Autodesk Inventor part; units mm, degrees
ref_plane "YZ Plane" through (0, 0, 0) normal (1, 0, 0) x (0, 1, 0)
ref_plane "XZ Plane" through (0, 0, 0) normal (0, 1, 0) x (-1, 0, 0)
ref_plane "XY Plane" through (0, 0, 0) normal (0, 0, 1) x (1, 0, 0)
sketch "Sketch1" plane through (0, 0, 0) normal (1, 0, 0) x (0, 1, 0)
  line L0 (95.25, -63.5) -> (7.9502, -63.5) construction
  arc A0 (95.25, -63.5) -> (127, -31.75) centre (95.25, -31.75) ccw construction
  circle A1 centre (104.9083, -202.0677) radius 25.4 construction
  circle A2 centre (104.9083, -202.0677) radius 14.2875
  circle A3 centre (154.8209, -171.8196) radius 25.4 construction
  circle A4 centre (154.8209, -171.8196) radius 14.2875
  circle A5 centre (250.0002, -47.5843) radius 22.225 construction
  circle A6 centre (250.0002, -47.5843) radius 25.4 construction
  circle A7 centre (250.0002, -47.5843) radius 14.2875
  circle A8 centre (154.8209, -171.8196) radius 22.225 construction
  circle A9 centre (104.9083, -202.0677) radius 22.225 construction
  circle A10 centre (25.4, -99.06) radius 25.4 construction
  circle A11 centre (25.4, -99.06) radius 23.8125 construction
  line L1 (25.4, -73.66) -> (25.4, -63.5) construction
  circle A12 centre (219.8086, -102.3786) radius 25.4 construction
  circle A13 centre (219.8086, -102.3786) radius 22.225 construction
  circle A14 centre (219.8086, -102.3786) radius 14.2875
  circle A15 centre (63.172, -79.375) radius 6.477 construction
  circle A16 centre (25.4, -99.06) radius 14.2875
  circle A17 centre (63.172, -79.375) radius 3.2512 construction
  circle A18 centre (166.1747, -221.0415) radius 3.2512 construction
  line L2 (219.8086, -102.3786) -> (154.8209, -171.8196) construction
  line L3 (154.8209, -171.8196) -> (104.9083, -202.0677) construction
  circle A19 centre (166.1747, -221.0415) radius 6.4262 construction
  circle A20 centre (63.172, -79.375) radius 6.35 construction
  circle A21 centre (25.4, -99.06) radius 22.225 construction
  line L4 (3.175, -99.06) -> (3.175, -68.2752) construction
  arc A22 (166.1747, -227.4677) -> (170.1786, -226.0679) centre (166.1747, -221.0415) ccw
  arc A23 (3.175, -99.06) -> (35.6756, -118.7669) centre (25.4, -99.06) ccw construction
  arc A24 (7.9502, -63.5) -> (3.175, -68.2752) centre (7.9502, -68.2752) ccw construction
  line L5 (232.868, -28.832) -> (267.1324, -66.3365) construction
  circle A25 centre (232.868, -28.832) radius 2.4257
  circle A26 centre (267.1324, -66.3365) radius 2.4257 construction
  circle A27 centre (232.868, -28.832) radius 6.35 construction
  circle A28 centre (267.1324, -66.3365) radius 6.35 construction
  line L6 (219.8086, -102.3786) -> (237.1646, -83.8332) construction
  line L7 (219.8086, -102.3786) -> (202.4526, -120.9239) construction
  circle A29 centre (237.1646, -83.8332) radius 2.4257 construction
  circle A30 centre (202.4526, -120.9239) radius 2.4257 construction
  circle A31 centre (172.1769, -153.2743) radius 2.4257 construction
  circle A32 centre (133.0985, -184.9838) radius 2.4257 construction
  arc A33 (83.3089, -196.8314) -> (103.7686, -224.2634) centre (104.9083, -202.0677) ccw
  circle A34 centre (9.525, -79.2321) radius 2.4257
  circle A35 centre (9.525, -79.2321) radius 6.35 construction
  line L8 (9.525, -79.2321) -> (41.275, -118.8879) construction
  circle A36 centre (41.275, -118.8879) radius 2.4257 construction
  circle A37 centre (41.275, -118.8879) radius 5.6007 construction
  line L9 (7.9502, -63.5) -> (95.25, -63.5) construction
  arc A38 (95.25, -63.5) -> (127, -31.75) centre (95.25, -31.75) ccw construction
  line L10 (166.1747, -227.4677) -> (103.7686, -224.2634)
  line L11 (104.9083, -202.0677) -> (83.1859, -215.2319) construction
  line L12 (127, -31.75) -> (127, -26.9595) construction
  circle A39 centre (133.0985, -184.9838) radius 5.6007 construction
  circle A40 centre (277.7476, -102.0288) radius 30 construction
  circle A41 centre (277.7476, -102.0288) radius 25.4 construction
  circle A42 centre (277.7476, -102.0288) radius 9.525
  circle A43 centre (219.8086, -102.3786) radius 19.05 construction
  circle A44 centre (227.4601, -139.7023) radius 19.05 construction
  circle A45 centre (227.4601, -139.7023) radius 14.2875
  line L13 (247.7482, -102.2099) -> (245.2082, -102.2252) construction
  line L14 (170.1786, -226.0679) -> (296.4391, -125.4942)
  arc A46 (296.4391, -125.4942) -> (303.3752, -86.4331) centre (277.7476, -102.0288) ccw
  circle A47 centre (219.8086, -102.3786) radius 30.48 construction
  circle A48 centre (277.7476, -102.0288) radius 30.48 construction
  circle A49 centre (248.6408, -79.4624) radius 3.81 construction
  line L15 (251.6519, -81.7968) -> (253.6592, -83.3531) construction
  line L16 (245.6582, -81.833) -> (243.6698, -83.4134) construction
  circle A50 centre (248.6408, -79.4624) radius 2.3812 construction
  circle A51 centre (248.9154, -124.945) radius 3.81 construction
  circle A52 centre (248.9154, -124.945) radius 2.3876 construction
  line L17 (251.898, -122.5744) -> (253.8865, -120.9939) construction
  line L18 (245.9043, -122.6105) -> (243.897, -121.0542) construction
  line L19 (248.6408, -75.6524) -> (248.6408, -72.9479) construction
  line L20 (219.8086, -102.3786) -> (219.8086, -88.0911) construction
  line L21 (131.7752, -22.1843) -> (250.0002, -22.1843)
  line L22 (271.6983, -34.3799) -> (303.3752, -86.4331)
  arc A53 (271.6983, -34.3799) -> (250.0002, -22.1843) centre (250.0002, -47.5843) ccw
  arc A54 (131.7752, -22.1843) -> (127, -26.9595) centre (131.7752, -26.9595) ccw
  circle A55 centre (146.08, -220.0775) radius 6.35 construction
  circle A56 centre (146.08, -220.0775) radius 2.4257
  circle A57 centre (253.6387, -151.4689) radius 6.35 construction
  circle A58 centre (253.6387, -151.4689) radius 2.4257
  circle A59 centre (209.9304, -186.285) radius 6.35 construction
  circle A60 centre (209.9304, -186.285) radius 2.4257
  circle A61 centre (123.7263, -57.0623) radius 6.35 construction
  circle A62 centre (123.7263, -57.0623) radius 2.4257
  circle A63 centre (281.6771, -62.9926) radius 6.35 construction
  circle A64 centre (281.6771, -62.9926) radius 2.4257
  line L23 (123.7263, -57.0623) -> (232.868, -28.832) construction
  line L24 (232.868, -28.832) -> (281.6771, -62.9926) construction
  line L25 (281.6771, -62.9926) -> (253.6387, -151.4689) construction
  line L26 (253.6387, -151.4689) -> (209.9304, -186.285) construction
  line L27 (209.9304, -186.285) -> (146.08, -220.0775) construction
  line L28 (146.08, -220.0775) -> (9.525, -79.2321) construction
  line L29 (123.7263, -57.0623) -> (9.525, -79.2321) construction
  line L30 (117.555, -55.5662) -> (83.3089, -196.8314)
  arc A65 (118.9802, -52.8436) -> (127, -26.9595) centre (94.4844, -31.0695) ccw
  arc A66 (118.9802, -52.8436) -> (117.555, -55.5662) centre (123.7263, -57.0623) ccw
  point P0 (180.2209, -171.8196)
  point P1 (172.6009, -221.0415)
  point P2 (104.9083, -227.4677)
  point P3 (127, -22.1843)
  point P4 (250.0002, -47.5843)
  point P5 (0, 0)
  point P6 (95.25, -63.5)
  dimension "d4" = 31.75
  dimension "d17" = 50.8
  dimension "d18" = 1.5875
  dimension "d21" = 12.954
  dimension "d22" = 28.575
  dimension "d23" = 6.5024
  dimension "d26" = 130.175
  dimension "d27" = 15.875
  dimension "d28" = 6.5024
  dimension "d29" = 143.1895
  dimension "d41" = 3.175
  dimension "d42" = 12.7
  dimension "d43" = 10.16
  dimension "d44" = 50.8
  dimension "d45" = 3.175
  dimension "d46" = 44.45
  dimension "d53" = 3.175
  dimension "d55" = 4.7752
  dimension "d59" = 4.8514
  dimension "d60" = 4.8514
  dimension "d68" = 4.8514
  dimension "d69" = 4.8514
  dimension "d70" = 4.8514
  dimension "d71" = 4.8514
  dimension "d72" = 4.8514
  dimension "d74" = 4.8514
  dimension "d75" = 3.175
  dimension "d86" = 7.62
  dimension "d88" = 3.175
  dimension "d90" = 58.3628
  dimension "d92" = 60
  dimension "d93" = 50.8
  dimension "d96" = 19.05
  dimension "d97" = 38.1
  dimension "d98" = 38.1
  dimension "d99" = 28.575
  dimension "d100" = 56.9248
  dimension "d101" = 2.54
  dimension "d102" = 60.96
  dimension "d103" = 60.96
  dimension "d104" = 7.62
  dimension "d105" = 2.54
  dimension "d106" = 4.7625
  dimension "d107" = 7.62
  dimension "d108" = 4.7752
  dimension "d109" = 2.54
  dimension "d111" = 2.7045
  dimension "d112" = 38.682
  dimension "d113" = 7.6515
  dimension "d114" = 202.0601
  dimension "d115" = 40.6423
  dimension "d116" = 37.3238
  dimension "d117" = 95.1077
  dimension "d118" = 57.939
  dimension "d119" = 62.8341
  dimension "d120" = 61.1075
  dimension "d121" = 250.0002
  dimension "d122" = 99.06
  dimension "d123" = 25.4
  dimension "d125" = 127
  dimension "d128" = 130.1236
  dimension "d129" = 232.868
  dimension "d130" = 4.7752
  dimension "d131" = 22.1843
extrude "Extrusion2" add sketch "Sketch1" along normal blind 4.7625 contours L10 A33 L30 A66 A65 A54 L21 A53 L22 A46 L14 A22
properties part number "INTK_001_PulleyCover" material "Polycarbonate, Clear"
Input: part model. Units: mm. Frame: model coordinates. Coordinates: 2 decimals unless noted, no trailing zeros. Loops run counter-clockwise (first coordinate to the right, second up) from the corner with the lowest first, then second, coordinate; pieces in that order, holes last.
Q1. Contact query for flat-ended pins moving along their axis: pin 1 (6 mm diameter, centred on y = 231, z = -151, fed in from +X); pin 2 (1.5 mm diameter, centred on x = 2, y = 276, fed in from -Z). Output: stop coordinate, or through.
Q2. Draft query along Z for faces 1 (the face through (0, 194, -123)), 2 (the face through (2.348, 279.254, -63.099)), 3 (the face through (2.348, 232.425, -176.485)), 4 (the face through (2.35, 125.85, -40.58)). Return one class per face: +Z half, -Z half, draft (parallel to the pull), parting line (faces both ways), or undercut.
Q3. Cut plane D-D (y = 157). Output: boundary loops of the cut face in (x, z), then the cut area to 3 significant figures.
Q4. Cut plane B-B (z = -174.5). Output: boundary loops of the cut face in (x, y), then the cut area to 3 significant figures.
Q5. Material intervals for line 1 (Y direction, x = 1.3, z = -58.5); line 2 (Z direction, x = 3.9, y = 254); line 3 (Y direction, x = 2.95, z = -184.5), sorted ascending.
Q6. Cut plane A-A (y = 224). Output: boundary loops of the cut face in (x, z).
Q7. Cut plane C-C (x = 2.55). Give the number of separate pieces and of enclosed holes in the cut face, then the cut area to 3 significant figures.
Working result:
1. pin 1: stops at x = 4.76
1. pin 2: stops at z = -142.37
2. face 1: draft
2. face 2: undercut
2. face 3: -Z half
2. face 4: undercut
3. outline: (0, -227) - (4.76, -227) - (4.76, -185.94) - (0, -185.94) - close; (0, -157.7) - (4.76, -157.7) - (4.76, -22.18) - (0, -22.18) - close
3. area: 841 mm2
4. outline: (0, 88.72) - (4.76, 88.72) - (4.76, 140.79) - (0, 140.79) - close; (0, 168.85) - (4.76, 168.85) - (4.76, 234.92) - (0, 234.92) - close
4. area: 563 mm2
5. line 1: y = 116.84 to 121.77, 125.68 to 240.78, 259.22 to 286.38
5. line 2: z = -159.3 to -153.87, -149.07 to -61.3, -33.87 to -22.5
5. line 3: y = 86.3 to 148.24, 161.4 to 208.29, 211.57 to 222.36
6. outline: (0, -183.2) - (4.76, -183.2) - (4.76, -153.56) - (0, -153.56) - close; (0, -125.84) - (4.76, -125.84) - (4.76, -116.04) - (0, -116.04) - close; (0, -88.72) - (4.76, -88.72) - (4.76, -22.18) - (0, -22.18) - close
7. separate pieces: 1
7. enclosed holes: 12
7. area: 29,100 mm2
